```python
from build123d import *

# Parameters (mm, degrees)
EXTRUDE1_DEPTH = 2.22
EXTRUDE6_DEPTH = 0.02
SKETCH2_R      = 0.25
EXTRUDE7_DEPTH = 2.5


with BuildPart() as part:
    # Sketch1 → Extrude1 (new body)
    with BuildSketch(Plane.XY):
        with BuildLine():
            Line((-6.39861095, 5.506998303), (-4.99861095, 5.506998303))
            ThreePointArc((-4.99861095, 5.506998303), (-3.725818744, 4.979790509), (-3.19861095, 3.706998303))
            Line((-3.19861095, 3.706998303), (-3.19861095, 3.006998303))
            ThreePointArc((-3.19861095, 3.006998303), (-3.725818744, 1.734206097), (-4.99861095, 1.206998303))
            Line((-4.99861095, 1.206998303), (-6.39861095, 1.206998303))
            ThreePointArc((-6.39861095, 1.206998303), (-7.671403156, 1.734206097), (-8.19861095, 3.006998303))
            Line((-8.19861095, 3.006998303), (-8.19861095, 3.706998303))
            ThreePointArc((-8.19861095, 3.706998303), (-7.671403156, 4.979790509), (-6.39861095, 5.506998303))
        make_face()
    extrude(amount=EXTRUDE1_DEPTH)

    # Sketch3 → Extrude6 (add)
    with BuildSketch(Plane.XY.offset(2.22)):
        with BuildLine():
            Line((-4.659129836, 4.836998303), (-7.799717656, 4.836998303))
            Line((-7.799717656, 4.836998303), (-7.757450007, 4.887488208))
            Line((-7.757450007, 4.887488208), (-7.674189251, 4.976998303))
            Line((-7.674189251, 4.976998303), (-4.664395148, 4.976998303))
            ThreePointArc((-4.664395148, 4.976998303), (-4.452263114, 4.889130337), (-4.364395148, 4.676998303))
            Line((-4.364395148, 4.676998303), (-4.364395148, 4.619148396))
            ThreePointArc((-4.364395148, 4.619148396), (-4.452263114, 4.407016361), (-4.664395148, 4.319148396))
            Line((-4.664395148, 4.319148396), (-6.560237828, 4.319148396))
            ThreePointArc((-6.560237828, 4.319148396), (-6.666303845, 4.275214413), (-6.710237828, 4.169148396))
            Line((-6.710237828, 4.169148396), (-6.710237828, 4.093148396))
            ThreePointArc((-6.710237828, 4.093148396), (-6.666303845, 3.987082379), (-6.560237828, 3.943148396))
            Line((-6.560237828, 3.943148396), (-4.664395148, 3.943148396))
            ThreePointArc((-4.664395148, 3.943148396), (-4.452263114, 3.85528043), (-4.364395148, 3.643148396))
            Line((-4.364395148, 3.643148396), (-4.364395148, 3.587148396))
            ThreePointArc((-4.364395148, 3.587148396), (-4.452263114, 3.375016361), (-4.664395148, 3.287148396))
            Line((-4.664395148, 3.287148396), (-6.560237828, 3.287148396))
            ThreePointArc((-6.560237828, 3.287148396), (-6.666303845, 3.243214413), (-6.710237828, 3.137148396))
            Line((-6.710237828, 3.137148396), (-6.710237828, 3.061148396))
            ThreePointArc((-6.710237828, 3.061148396), (-6.666303845, 2.955082379), (-6.560237828, 2.911148396))
            Line((-6.560237828, 2.911148396), (-4.664395148, 2.911148396))
            ThreePointArc((-4.664395148, 2.911148396), (-4.452263114, 2.82328043), (-4.364395148, 2.611148396))
            Line((-4.364395148, 2.611148396), (-4.364395148, 2.555148396))
            ThreePointArc((-4.364395148, 2.555148396), (-4.452263114, 2.343016361), (-4.664395148, 2.255148396))
            Line((-4.664395148, 2.255148396), (-6.560237828, 2.255148396))
            ThreePointArc((-6.560237828, 2.255148396), (-6.666303845, 2.211214413), (-6.710237828, 2.105148396))
            Line((-6.710237828, 2.105148396), (-6.710237828, 2.024997149))
            ThreePointArc((-6.710237828, 2.024997149), (-6.666303845, 1.918931132), (-6.560237828, 1.874997149))
            Line((-6.560237828, 1.874997149), (-3.599120547, 1.874997149))
            Line((-3.599120547, 1.874997149), (-3.725818744, 1.734206097))
            Line((-3.725818744, 1.734206097), (-6.554972516, 1.734206097))
            ThreePointArc((-6.554972516, 1.734206097), (-6.767104551, 1.822074063), (-6.854972516, 2.034206097))
            Line((-6.854972516, 2.034206097), (-6.854972516, 2.093703593))
            ThreePointArc((-6.854972516, 2.093703593), (-6.767104551, 2.305835627), (-6.554972516, 2.393703593))
            Line((-6.554972516, 2.393703593), (-4.659129836, 2.393703593))
            ThreePointArc((-4.659129836, 2.393703593), (-4.553063819, 2.437637576), (-4.509129836, 2.543703593))
            Line((-4.509129836, 2.543703593), (-4.509129836, 2.619703593))
            ThreePointArc((-4.509129836, 2.619703593), (-4.553063819, 2.72576961), (-4.659129836, 2.769703593))
            Line((-4.659129836, 2.769703593), (-6.554972516, 2.769703593))
            ThreePointArc((-6.554972516, 2.769703593), (-6.767104551, 2.857571559), (-6.854972516, 3.069703593))
            Line((-6.854972516, 3.069703593), (-6.854972516, 3.125703593))
            ThreePointArc((-6.854972516, 3.125703593), (-6.767104551, 3.337835627), (-6.554972516, 3.425703593))
            Line((-6.554972516, 3.425703593), (-4.659129836, 3.425703593))
            ThreePointArc((-4.659129836, 3.425703593), (-4.553063819, 3.469637576), (-4.509129836, 3.575703593))
            Line((-4.509129836, 3.575703593), (-4.509129836, 3.651703593))
            ThreePointArc((-4.509129836, 3.651703593), (-4.553063819, 3.75776961), (-4.659129836, 3.801703593))
            Line((-4.659129836, 3.801703593), (-6.554972516, 3.801703593))
            ThreePointArc((-6.554972516, 3.801703593), (-6.767104551, 3.889571559), (-6.854972516, 4.101703593))
            Line((-6.854972516, 4.101703593), (-6.854972516, 4.157703593))
            ThreePointArc((-6.854972516, 4.157703593), (-6.767104551, 4.369835627), (-6.554972516, 4.457703593))
            Line((-6.554972516, 4.457703593), (-4.659129836, 4.457703593))
            ThreePointArc((-4.659129836, 4.457703593), (-4.553063819, 4.501637576), (-4.509129836, 4.607703593))
            Line((-4.509129836, 4.607703593), (-4.509129836, 4.686998303))
            ThreePointArc((-4.509129836, 4.686998303), (-4.553063819, 4.79306432), (-4.659129836, 4.836998303))
        make_face()
    extrude(amount=EXTRUDE6_DEPTH)

    # Sketch2 → Extrude7 (add)
    with BuildSketch(Plane(origin=(0, 0, 0), x_dir=(-1, 0, 0), z_dir=(0, 0, -1))):
        with Locations(Location((4.07361095, 3.356998303, 0), (0, 0, 180))):
            Circle(SKETCH2_R)
        with Locations(Location((7.32361095, 3.356998303, 0), (0, 0, 180))):
            Circle(SKETCH2_R)
    extrude(amount=EXTRUDE7_DEPTH)


solid = part.part
```
Verification items for the finished model (mm, model axes). A direction names the side the tool comes from. Round coordinates to 2 decimals unless told otherwise and drop trailing zeros. Order: outer loops, then holes, each group sorted by start corner. A loop starts at its lowest first (then second) coordinate and runs counter-clockwise, first axis right, second up.
1) Cross-section at A-A, the plane z = 0.15. Record the cut outline in (x, y), plus the area to 3 significant figures.
Geometry says:
outline: (-8.2, 3.01) arc R1.8 ccw to (-6.4, 1.21) - (-5, 1.21) arc R1.8 ccw to (-3.2, 3.01) - (-3.2, 3.71) arc R1.8 ccw to (-5, 5.51) - (-6.4, 5.51) arc R1.8 ccw to (-8.2, 3.71) - close
area: 18.7 mm2
2) Tool access check on faces 1 (the flat face through (-4, 4, 2.22)), 2 (the cylindrical face through (-3.71, 1.75, 1.09)), 3 (the flat face through (-7, 3, 2.22)). Record the directions out of +Z, -Z, +X, -X, +Y, -Y that give a thin tool (end or side, any length) a straight path to the whole face; none if there is none.
Geometry says:
face 1: +Z, +X
face 2: +Z, -Z, +X, -Y
face 3: +Z, -X
3) Depth check by flat-ended pin: pin 1 (1 mm diameter, centred on x = -6, y = 4.5, fed in from -Z). Enter the tip coordinate at first touch or a pass-through.
Geometry says:
pin 1: stops at z = 0
4) Cross-section at C-C, the plane x = -4.05. Record the cut outline in (y, z) (3 decimals), plus the area to 3 significant figures.
Geometry says:
outline: (1.477, 0) - (3.108, 0) - (3.108, -2.5) - (3.606, -2.5) - (3.606, 0) - (5.237, 0) - (5.237, 2.22) - (1.875, 2.22) - (1.875, 2.24) - (1.734, 2.24) - (1.734, 2.22) - (1.477, 2.22) - close
area: 9.59 mm2
5) Material ranges on line 1 (Z direction, x = -6.55, y = 4.7); line 2 (X direction, y = 1.85, z = 0.9); line 3 (Z direction, x = -7.2, y = 3.35), recorded low to high.
Geometry says:
line 1: z = 0 to 2.22
line 2: x = -7.78 to -3.62
line 3: z = -2.5 to 2.22
6) Cross-section at D-D, the plane z = -1.4. Record the cut outline in (x, y).
Geometry says:
outline: circle Ø0.5 at (-7.32, 3.36); circle Ø0.5 at (-4.07, 3.36)
